```python
from build123d import *

# Parameters (mm, degrees)
SKETCH008_W   = 17
SKETCH008_H   = 14.5
SKETCH008_W_2 = 16
SKETCH008_H_2 = 17.3
PAD002_DEPTH  = 3
FILLET_R      = 3
FILLET004_R   = 1


with BuildPart() as part:
    # Sketch008 → Pad002 (new body)
    with BuildSketch(Plane.YZ.offset(93)):
        Polygon((-42.5, 3), (-42.5, 0), (-22.5, 0), (-22.5, 3), (0, 3), (0, 11), (-3, 11), (-3, 21.2), (0, 21.2), (0, 29.2), (-22.5, 29.2), (-22.5, 32.2), (-42.5, 32.2), (-42.5, 29.2), (-65, 29.2), (-65, 21.2), (-62, 21.2), (-62, 11), (-65, 11), (-65, 3), align=None)
        with Locations((-50, 17.25)):
            Rectangle(SKETCH008_W, SKETCH008_H, mode=Mode.SUBTRACT)
        with Locations((-13, 18.65)):
            Rectangle(SKETCH008_W_2, SKETCH008_H_2, mode=Mode.SUBTRACT)
        with Locations((-31.4, 18.65)):
            Rectangle(SKETCH008_W_2, SKETCH008_H_2, mode=Mode.SUBTRACT)
    extrude(amount=-PAD002_DEPTH)

    # Fillet
    fillet_edges = [part.edges().sort_by_distance(p)[0] for p in [
        (91.5, -23.4, 10),
        (91.5, -5, 10),
        (91.5, -5, 27.3),
        (91.5, -23.4, 27.3),
        (91.5, -21, 10),
        (91.5, -39.4, 10),
        (91.5, -21, 27.3),
        (91.5, -39.4, 27.3),
    ]]
    fillet(fillet_edges, radius=FILLET_R)

    # Fillet004
    fillet004_edges = [part.edges().sort_by_distance(p)[0] for p in [
        (91.5, -58.5, 10),
        (91.5, -58.5, 24.5),
        (91.5, -41.5, 24.5),
        (91.5, -41.5, 10),
    ]]
    fillet(fillet004_edges, radius=FILLET004_R)


solid = part.part
```
Read the model definition and answer for the solid it produces. Units are mm, in the model's axes. A direction names the side the tool comes from. Round coordinates to 2 decimals unless told otherwise and drop trailing zeros. Write each loop counter-clockwise with the first axis right and the second up, starting at its lowest first coordinate (ties: lowest second). Pieces come first, ordered by that corner, then holes. Notation, with made-up numbers: M 58,14.5 L 70,14.5 A15 ccw 70,34.5 Z; hole C -15,46 d6. An arc over 180 degrees is marked long. One line per item, written item: value.
Q1. Find section A-A on y = -9. Write down the section's boundary in (x, z).
Data:
outline: M 90,3 L 93,3 L 93,10 L 90,10 Z; M 90,27.3 L 93,27.3 L 93,29.2 L 90,29.2 Z
Q2. Find section D-D on x = 90.55. Count the separate pieces of the cut face and the enclosed holes in it, plus the area to 3 significant figures.
Data:
separate pieces: 1
enclosed holes: 3
area: 978 mm2
Q3. Flat-ended cylindrical pins translate along their axes: pin 1 Ø1.5 at (x, z) = (92, 1.5) entering from +Y; pin 2 Ø0.9 at (x, y) = (92, -32) entering from -Z; pin 3 Ø1.5 at (x, y) = (92, -1) entering from +Z; pin 4 Ø0.9 at (x, z) = (91, 20) entering from -Y. Find the tip coordinate at first contact, or state that the pin passes through.
Data:
pin 1: y = -22.5
pin 2: z = 0
pin 3: z = 29.2
pin 4: y = -62
Q4. Straight lines are drawn through the part: line 1 (Y direction, x = 92.55, z = 22.5); line 2 (Y direction, x = 91.35, z = 14); line 3 (Z direction, x = 91.55, y = -10). For each, find the intervals that lie inside material, in ascending order. Write a range as [from, to].
Data:
line 1: [-65, -58.5], [-41.5, -39.4], [-23.4, -21], [-5, 0]
line 2: [-62, -58.5], [-41.5, -39.4], [-23.4, -21], [-5, -3]
line 3: [3, 10], [27.3, 29.2]
Q5. Find section C-C on y = -51.5. Write down the section's boundary in (x, z), plus the area to 3 significant figures.
Data:
outline: M 90,3 L 93,3 L 93,10 L 90,10 Z; M 90,24.5 L 93,24.5 L 93,29.2 L 90,29.2 Z
area: 35.1 mm2
Q6. For a pull along Y with two mould halves and no side action, classify faces 5 (the flat face through (92, -50, 24.5)), 6 (the flat face through (92, -31, 10)), 7 (the flat face through (92, -65, 7)), 8 (the flat face through (92, 0, 25)) as +Y half, -Y half, draft (parallel to the pull), parting line (faces both ways), or undercut.
Data:
face 5: undercut
face 6: undercut
face 7: -Y half
face 8: +Y half
Q7. Find section B-B on z = 18. Write down the section's boundary in (x, y).
Data:
outline: M 90,-62 L 93,-62 L 93,-58.5 L 90,-58.5 Z; M 90,-41.5 L 93,-41.5 L 93,-39.4 L 90,-39.4 Z; M 90,-23.4 L 93,-23.4 L 93,-21 L 90,-21 Z; M 90,-5 L 93,-5 L 93,-3 L 90,-3 Z
Q8. Which of the six approach directions +Z, -Z, +X, -X, +Y, -Y give full straight-line access (tool end or side, diameter ignored) to faces 1 (the flat face through (92, -1, 11)), 2 (the flat face through (92, -39.4, 19)), 3 (the flat face through (92, -22.5, 1)), 4 (the flat face through (92, -54, 29.2))?
Data:
face 1: +X, -X, +Y
face 2: +X, -X
face 3: -Z, +X, -X, +Y
face 4: +Z, +X, -X, -Y
